Design review of the part built by this model. Coordinates are the model's own, in mm. Face numbers are marked on the shaded views. A direction names the side the tool comes from. Coordinates: 2 decimals unless noted, no trailing zeros. Write each loop counter-clockwise with the first axis right and the second up, starting at its lowest first coordinate (ties: lowest second). Pieces come first, ordered by that corner, then holes.
```python
from build123d import *

# Parameters (mm, degrees)
SKETCH1_W               = 90
SKETCH1_H               = 40
BOSS_EXTRUDE1_DEPTH     = 10
CUT_EXTRUDE1_DEPTH      = 67
CUT_EXTRUDE1_DEPTH_BACK = 33
SKETCH2_R               = 2.75
CUT_EXTRUDE2_DEPTH      = 56
CUT_EXTRUDE2_DEPTH_BACK = 35
SKETCH2_4_R             = 2.75
SKETCH2_5_R             = 5
CUT_EXTRUDE3_DEPTH      = 5.4
SKETCH2_6_R             = 5
CUT_EXTRUDE4_DEPTH      = 5.4


with BuildPart() as part:
    # Sketch1 → Boss-Extrude1 (new body)
    with BuildSketch(Plane.XY):
        with Locations((-1.816720257, -1.54340836)):
            Rectangle(SKETCH1_W, SKETCH1_H)
    extrude(amount=BOSS_EXTRUDE1_DEPTH)

    # Sketch2 → Cut-Extrude1 (cut, two sides: drawn at the far end of the back side and taken through both)
    with BuildSketch(Plane.XY.offset(10).offset(-CUT_EXTRUDE1_DEPTH_BACK)):
        with Locations((-39.816720257, -1.54340836)):
            Circle(SKETCH2_R)
    extrude(amount=CUT_EXTRUDE1_DEPTH + CUT_EXTRUDE1_DEPTH_BACK, mode=Mode.SUBTRACT)

    # Sketch2<4> → Cut-Extrude2 (cut, two sides: drawn at the far end of the back side and taken through both)
    with BuildSketch(Plane.XY.offset(10).offset(-CUT_EXTRUDE2_DEPTH_BACK)):
        with Locations((36.183279743, -1.54340836)):
            Circle(SKETCH2_4_R)
    extrude(amount=CUT_EXTRUDE2_DEPTH + CUT_EXTRUDE2_DEPTH_BACK, mode=Mode.SUBTRACT)

    # Sketch2<5> → Cut-Extrude3 (cut)
    with BuildSketch(Plane.XY.offset(10)):
        with Locations((-39.816720257, -1.54340836)):
            Circle(SKETCH2_5_R)
    extrude(amount=-CUT_EXTRUDE3_DEPTH, mode=Mode.SUBTRACT)

    # Sketch2<6> → Cut-Extrude4 (cut)
    with BuildSketch(Plane.XY.offset(10)):
        with Locations((36.183279743, -1.54340836)):
            Circle(SKETCH2_6_R)
    extrude(amount=-CUT_EXTRUDE4_DEPTH, mode=Mode.SUBTRACT)


solid = part.part
```
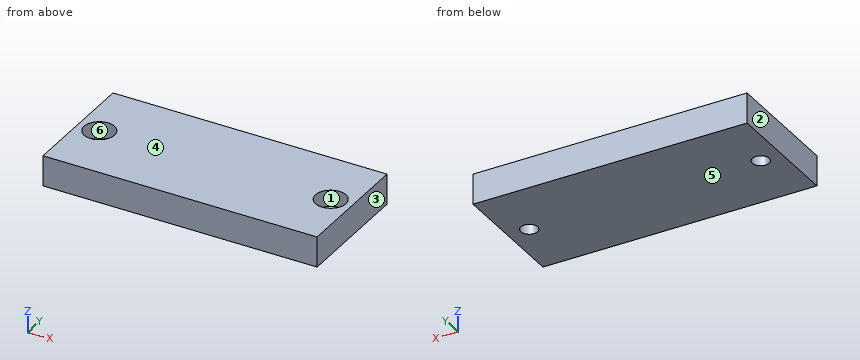
(1) Insertion check: pin 1 Ø8 at (x, y) = (-39.82, -1.54) entering from +Z. The pin has a flat end and moves straight along its axis. Give the tip position at first contact, or say it passes through.
(2) Wall thickness on line 1 (X direction, y = 0, z = 5); line 2 (X direction, y = -3, z = 4.5); line 3 (Y direction, x = 37, z = 9): over which ranges is each line inside the solid? List them lowest first.
(3) Consider section C-C (z = 8.25). Give the boundary of the cut face in (x, y), plus the area to 3 significant figures.
(4) Mouldability with a two-part tool opening along X and no side actions: class the marked faces 1, 2, 3 and 4 as +X half, -X half, draft (parallel to the pull), parting line (faces both ways), or undercut.
(5) Consider section B-B (x = -41). Give the boundary of the cut face in (y, z).
(6) For the marked faces 5 and 6, list the 3-axis set-ups (+Z, -Z, +X, -X, +Y, -Y) from which the entire face can be reached by the end or side of a thin tool; tool diameter is ignored.
(7) Consider section A-A (y = 0). Give the boundary of the cut face in (x, z), plus the area to 3 significant figures.
Results:
1. pin 1: stops at z = 4.6
2. line 1: x = -46.82 to -44.57, -35.06 to 31.43, 40.94 to 43.18
2. line 2: x = -46.82 to -42.15, -37.48 to 33.85, 38.52 to 43.18
2. line 3: y = -21.54 to -6.48, 3.39 to 18.46
3. outline: (-46.82, -21.54) - (43.18, -21.54) - (43.18, 18.46) - (-46.82, 18.46) - close; hole circle Ø10 at (-39.82, -1.54); hole circle Ø10 at (36.18, -1.54)
3. area: 3,440 mm2
4. face 1: undercut
4. face 2: -X half
4. face 3: +X half
4. face 4: draft
5. outline: (-21.54, 0) - (-4.03, 0) - (-4.03, 4.6) - (-6.4, 4.6) - (-6.4, 10) - (-21.54, 10) - close; (0.94, 0) - (18.46, 0) - (18.46, 10) - (3.31, 10) - (3.31, 4.6) - (0.94, 4.6) - close
6. face 5: -Z, +X, -X, +Y, -Y
6. face 6: +Z
7. outline: (-46.82, 0) - (-42.09, 0) - (-42.09, 4.6) - (-44.57, 4.6) - (-44.57, 10) - (-46.82, 10) - close; (-37.54, 0) - (33.91, 0) - (33.91, 4.6) - (31.43, 4.6) - (31.43, 10) - (-35.06, 10) - (-35.06, 4.6) - (-37.54, 4.6) - close; (38.46, 0) - (43.18, 0) - (43.18, 10) - (40.94, 10) - (40.94, 4.6) - (38.46, 4.6) - close
7. area: 755 mm2
